Autodesk Inventor part; units mm, degrees
ref_plane "YZ Plane" through (0, 0, 0) normal (1, 0, 0) x (0, 1, 0)
ref_plane "XZ Plane" through (0, 0, 0) normal (0, 1, 0) x (-1, 0, 0)
ref_plane "XY Plane" through (0, 0, 0) normal (0, 0, 1) x (1, 0, 0)
sketch "Sketch1" plane through (0, 0, 0) normal (0, 0, 1) x (1, 0, 0)
  circle A0 centre (0, 0) radius 2.3241
  circle A1 centre (0, 0) radius 11.5062
  line L0 (0, 0) -> (0, 6.35)
  line L1 (0, 6.35) -> (1.4708, 6.35)
  line L2 (1.4708, 6.35) -> (9.5953, 6.35)
  line L3 (0, 6.35) -> (0, 19.05)
  line L4 (0, 19.05) -> (-6.35, 19.05)
  line L5 (-6.35, 19.05) -> (0, 6.35)
  line L6 (9.5953, 6.35) -> (0, 19.05)
  line L7 (0, 6.35) -> (-35.4663, 6.35)
  circle A2 centre (0, 0) radius 19.05
  line L8 (-30.5707, -30.0948) -> (-7.7493, -41.2459)
  circle A3 centre (4.7977, -18.436) radius 2.3241
  circle A4 centre (4.7977, -18.436) radius 4.7625
  line L9 (4.7977, -18.436) -> (-17.7887, -6.8164)
  circle A5 centre (-17.7887, -6.8164) radius 2.3241
  circle A6 centre (-17.7887, -6.8164) radius 4.7625
  line L10 (0, 6.35) -> (-19.7319, -2.4684)
  line L11 (9.5953, 6.35) -> (0, -11.5062)
  line L12 (0, -11.5062) -> (-17.7693, -11.5789)
  dimension "d0" = 4.6482
  dimension "d1" = 23.0124
  dimension "d2" = 6.35
  dimension "d3" = 12.7
  dimension "d4" = 6.35
  dimension "d5" = 25.4
  dimension "d6" = 4.6482
  dimension "d7" = 9.525
  dimension "d8" = 25.4
  dimension "d9" = 4.6482
  dimension "d10" = 9.525
extrude "Extrusion1" add sketch "Sketch1" along normal blind 6.35 contours L1 L2 L11 A1 L10 | L5 A1 L3 | L3 A1 L6 L2 L1 | L3 L6 A1 | A1 L5 A2 L3 | A1 L12 L9 A6 A2 L10 | A2 L5 L4 | A2 A6 L10 | L12 A2 A6 L9 | A6 L9 A5 A2 | A2 A5 A6 | A6 A2 A5 L9 | L12 A6 A2
properties part number "Goal Jaw Tooth"
Design review of the part built by this model. Coordinates are the model's own, in mm. A direction names the side the tool comes from. Give positions to 0.01 mm unless a question says otherwise; leave off trailing zeros. Write each loop counter-clockwise with the first axis right and the second up, starting at its lowest first coordinate (ties: lowest second). Pieces come first, ordered by that corner, then holes. Notation, with made-up numbers: M -8.75,38.5 L 47.25,38.5 A19 cw 47.25,47.5 Z; hole C 75.25,-29 d3. An arc over 180 degrees is marked long. Return JSON: item names as keys, results as strings. Group by question number.
Item 1: Clearance check with flat-ended pins moving along their axes: pin 1 Ø12 at (x, y) = (-13, 8.5) entering from +Z; pin 2 Ø3 at (x, z) = (-5.5, 4) entering from -Y. State where each tip first meets the part, or that it passes through.
Item 2: The part is to be moulded in two halves that separate along Y. For faces 3 (the flat face through (-9.73, 2, 3.13)), 4 (the flat face through (4.865, -2.453, 3.131)), 5 (the flat face through (4.865, 12.611, 3.131)), say which applies: pulls with the +Y half, pulls with the -Y half, needs draft (parallel to the pull), parting line crosses it, or undercut.
Item 3: Take a section at C-C (x = -15). Give the boundary of the cut face in (y, z), plus the area to 3 significant figures.
Item 4: Take a section at B-B (y = 0). Give the boundary of the cut face in (x, z), plus the area to 4 significant figures.
Item 5: Take a section at A-A (z = 4.25). Count the separate pieces of the cut face and the enclosed holes in it, plus the area to 3 significant figures.
Item 6: Wall thickness on line 1 along Y through (x, z) = (-5.5, 3.75); line 2 along Y through (x, z) = (2, 1.5); line 3 along X through (y, z) = (0, 4): over which ranges is each line inside the solid? List them lowest first.
Item 7: Tool access review of faces 1 (the flat face through (-3.22, 12.79, 3.13)), 2 (the flat face through (-3, 1, 0)): name each direction out of +Z, -Z, +X, -X, +Y, -Y from which nothing blocks a thin tool from reaching the whole face with its end or side.
Item 8: Take a section at D-D (y = 5). Give the boundary of the cut face in (x, z).
Return value:
{
 "1": {"pin 1": "passes through", "pin 2": "stops at y = -11.53"},
 "2": {"face 3": "undercut", "face 4": "pulls with the -Y half", "face 5": "pulls with the +Y half"},
 "3": {"outline": "M -11.57,0 L -0.35,0 L -0.35,6.35 L -11.57,6.35 Z", "area": "71.2 mm2"},
 "4": {"outline": "M -14.21,0 L -2.32,0 L -2.32,6.35 L -14.21,6.35 Z; M 2.32,0 L 6.18,0 L 6.18,6.35 L 2.32,6.35 Z", "area": "100.0 mm2"},
 "5": {"separate pieces": "1", "enclosed holes": "2", "area": "436 mm2"},
 "6": {"line 1": "y = -11.53 to 3.89, 17.35 to 19.05", "line 2": "y = -7.78 to -1.18, 1.18 to 16.4", "line 3": "x = -14.21 to -2.32, 2.32 to 6.18"},
 "7": {"face 1": "+Z, -Z, -X", "face 2": "-Z, +X, -X, +Y, -Y"},
 "8": {"outline": "M -3.02,0 L 8.87,0 L 8.87,6.35 L -3.02,6.35 Z"}
}
